```python
from build123d import *

# Parameters (mm, degrees)
SKETCH1_W                  = 254
SKETCH1_H                  = 254
SKETCH1_R                  = 10.16
SKETCH1_R_2                = 14.2875
BOSS_EXTRUDE2_DEPTH        = 6.35
F_9_0_196_DIAMETER_HOLE1_D = 4.9784


with BuildPart() as part:
    # Sketch1 → Boss-Extrude2 (new body)
    with BuildSketch(Plane.XY):
        Rectangle(SKETCH1_W, SKETCH1_H)
        with Locations((-41.221968309, 29.688201844)):
            Circle(SKETCH1_R, mode=Mode.SUBTRACT)
        with Locations((0, 49.5808)):
            Circle(SKETCH1_R_2, mode=Mode.SUBTRACT)
        Circle(SKETCH1_R_2, mode=Mode.SUBTRACT)
        with Locations((41.221968309, 29.688201844)):
            Circle(SKETCH1_R, mode=Mode.SUBTRACT)
    extrude(amount=BOSS_EXTRUDE2_DEPTH)

    # #9 (0.196) Diameter Hole1 (through all)
    with Locations(Plane(origin=(0, 0, 0), x_dir=(-1, 0, 0), z_dir=(0, 0, -1))):
        with Locations((-98.782817332, 98.782817332), (-52.261145976, 52.563877931), (-30.182790642, 6.812525757), (30.182790642, 6.812525757), (52.261145976, 52.563877931), (98.782817332, 98.782817332), (98.782817332, -98.782817332), (-98.782817332, -98.782817332), (-82.55, 74.9808), (-82.55, 24.1808), (82.55, 74.9808), (82.55, 24.1808)):
            Hole(F_9_0_196_DIAMETER_HOLE1_D / 2)


solid = part.part
```
Source: CAD feature listing. Evaluate the final solid. Frame: model axes, mm. Coordinates: 2 decimals unless noted, no trailing zeros. Write each loop counter-clockwise with the first axis right and the second up, starting at its lowest first coordinate (ties: lowest second). Pieces come first, ordered by that corner, then holes. Notation, with made-up numbers: M 14,24 L 72,24 A26 cw 72,49 Z; hole C 89,68.5 d11. An arc over 180 degrees is marked long. Answer as a JSON object with one key per item and string values.
1. Cut plane A-A on y = 0. Output: boundary loops of the cut face in (x, z), plus the area to 3 significant figures.
Evaluation:
{"outline": "M -127,0 L -14.29,0 L -14.29,6.35 L -127,6.35 Z; M 14.29,0 L 127,0 L 127,6.35 L 14.29,6.35 Z", "area": "1,430 mm^2"}
2. Ray query, L1, parallel to Y at x = 82.55, z = 3.75; L2, parallel to X at y = 29, z = 3.25; L3, parallel to Y at x = -40.5, z = 3.75. Return the intervals inside material, ascending.
Evaluation:
{"L1": "-127 to 21.69, 26.67 to 72.49, 77.47 to 127", "L2": "-127 to -51.36, -31.09 to 31.09, 51.36 to 127", "L3": "-127 to 19.55, 39.82 to 127"}
3. Cut plane C-C on z = 2.75. State how many separate pieces and enclosed holes the cut face has, plus the area to 3 significant figures.
Evaluation:
{"separate pieces": "1", "enclosed holes": "16", "area": "62,400 mm^2"}
4. Draft query along X for faces 1 (the flat face through (127, -2, 3)), 2 (the cylindrical face through (50.61, 25.8, 3.13)), 3 (the flat face through (-2, -26, 6.35)), 4 (the flat face through (-127, -2, 3)). Return one class per face: released by +X, released by -X, zero draft, split by the parting line, or undercut.
Evaluation:
{"face 1": "released by +X", "face 2": "undercut", "face 3": "zero draft", "face 4": "released by -X"}
5. Cut plane B-B on x = 0. Output: boundary loops of the cut face in (y, z), plus the area to 3 significant figures.
Evaluation:
{"outline": "M -127,0 L -14.29,0 L -14.29,6.35 L -127,6.35 Z; M 14.29,0 L 35.29,0 L 35.29,6.35 L 14.29,6.35 Z; M 63.87,0 L 127,0 L 127,6.35 L 63.87,6.35 Z", "area": "1,250 mm^2"}
